Build history of the part. All positions in model axes, mm. A direction names the side the tool comes from. Round coordinates to 2 decimals unless told otherwise and drop trailing zeros. Write each loop counter-clockwise with the first axis right and the second up, starting at its lowest first coordinate (ties: lowest second). Pieces come first, ordered by that corner, then holes. Notation, with made-up numbers: (22, 11.5) - (78, 11.5) arc R31 cw to (78, 42.5) - close; hole circle Ø9 at (11, 6). An arc over 180 degrees is marked (long way). One line per question, with ' | ' between items.
Autodesk Inventor part; units mm, degrees
ref_plane "YZ Plane" through (0, 0, 0) normal (1, 0, 0) x (0, 1, 0)
ref_plane "XZ Plane" through (0, 0, 0) normal (0, 1, 0) x (-1, 0, 0)
ref_plane "XY Plane" through (0, 0, 0) normal (0, 0, 1) x (1, 0, 0)
sketch "Sketch1" plane through (0, 0, 0) normal (0, 0, 1) x (1, 0, 0)
  circle A0 centre (0, 0) radius 12.7
  dimension "d0" = 25.4
extrude "Extrusion1" add sketch "Sketch1" along normal mid plane 107.6
sketch "Sketch2" plane through (0, 0, 0) normal (0, 1, 0) x (-1, 0, 0)
  circle A0 centre (0, 0) radius 9.525
  dimension "d3" = 19.05
extrude "Extrusion2" add sketch "Sketch2" along normal blind 53.8
shell "Shell1" thickness 1.65 removed faces 3 at (2.8113, 53.8, 0.0442) at (-3.6254, -0.9542, 53.8) at (-3.6254, -0.9542, -53.8)
properties part number "ASME BPE - RED TEE-25.4-19.05" material "Stainless Steel, 316L"
Q1. Saw through at A-A, the plane y = 0. List the corners of the cut face in (x, z).
Found:
outline: (-12.7, -53.8) - (-11.05, -53.8) - (-11.05, 53.8) - (-12.7, 53.8) - close; (11.05, -53.8) - (12.7, -53.8) - (12.7, 53.8) - (11.05, 53.8) - close
Q2. Saw through at B-B, the plane x = 0. List the corners of the cut face in (y, z) (3 decimals).
Found:
outline: (-12.7, -53.8) - (-11.05, -53.8) - (-11.05, 53.8) - (-12.7, 53.8) - close; (11.05, -53.8) - (12.7, -53.8) - (12.7, -9.525) - (53.8, -9.525) - (53.8, -7.875) - (11.05, -7.875) - close; (11.05, 7.875) - (53.8, 7.875) - (53.8, 9.525) - (12.7, 9.525) - (12.7, 53.8) - (11.05, 53.8) - close
Q3. Which spindle directions (+Z, -Z, +X, -X, +Y, -Y) get a long thin tool onto all of the face, cutting with end or side? Do faces 1 (the cylindrical face through (9.516, 30.782, -0.419)), 2 (the flat face through (4, 53.8, 7)). Say none if no direction does.
Found:
face 1: +Y | face 2: +Z, -Z, +X, -X, +Y
Q4. Saw through at C-C, the plane z = 0. List the corners of the cut face in (x, y) (3 decimals), then the cut area to 3 significant figures.
Found:
outline: (-9.525, 8.4) arc R12.7 ccw (long way) to (9.525, 8.4) - (9.525, 53.8) - (7.875, 53.8) - (7.875, 7.752) arc R11.05 cw (long way) to (-7.875, 7.752) - (-7.875, 53.8) - (-9.525, 53.8) - close | area: 242 mm^2
Q5. Drill centre lines: L1, parallel to Z at x = 0, y = 35 (3 decimals); L2, parallel to Y at x = 0, z = -23. Where is each one in solid material? Low to high. Write a range as from..to.
Found:
L1: -9.525..-7.875, 7.875..9.525 | L2: -12.7..-11.05, 11.05..12.7
Q6. Pull direction X, two halves, no side cores. Call faces 3 (the cylindrical face through (-1.438, -10.956, -0.753)), 4 (the cylindrical face through (7.867, 30.453, -0.346)), 5 (the flat face through (-1, -11.2, -53.8)), 6 (the cylindrical face through (-1.653, -12.592, -0.753)): +X half, -X half, draft (parallel to the pull), parting line (faces both ways), or undercut.
Found:
face 3: undercut | face 4: undercut | face 5: draft | face 6: parting line
Q7. Drop flat-ended pins along their axis: pin 1 (3 mm diameter, centred on x = -4, z = -8.5, fed in from -Y); pin 2 (3 mm diameter, centred on x = 3, y = 45.5, fed in from -Z); pin 3 (9.5 mm diameter, centred on x = 0, z = 0, fed in from +Y). Give the stop position or say it passes through.
Found:
pin 1: y = -12.45 | pin 2: z = -9.41 | pin 3: y = -9.98
Q8. Saw through at D-D, the plane y = 45. List the corners of the cut face in (x, z) (3 decimals).
Found:
outline: circle Ø19.05 at (0, 0); hole circle Ø15.75 at (0, 0)
